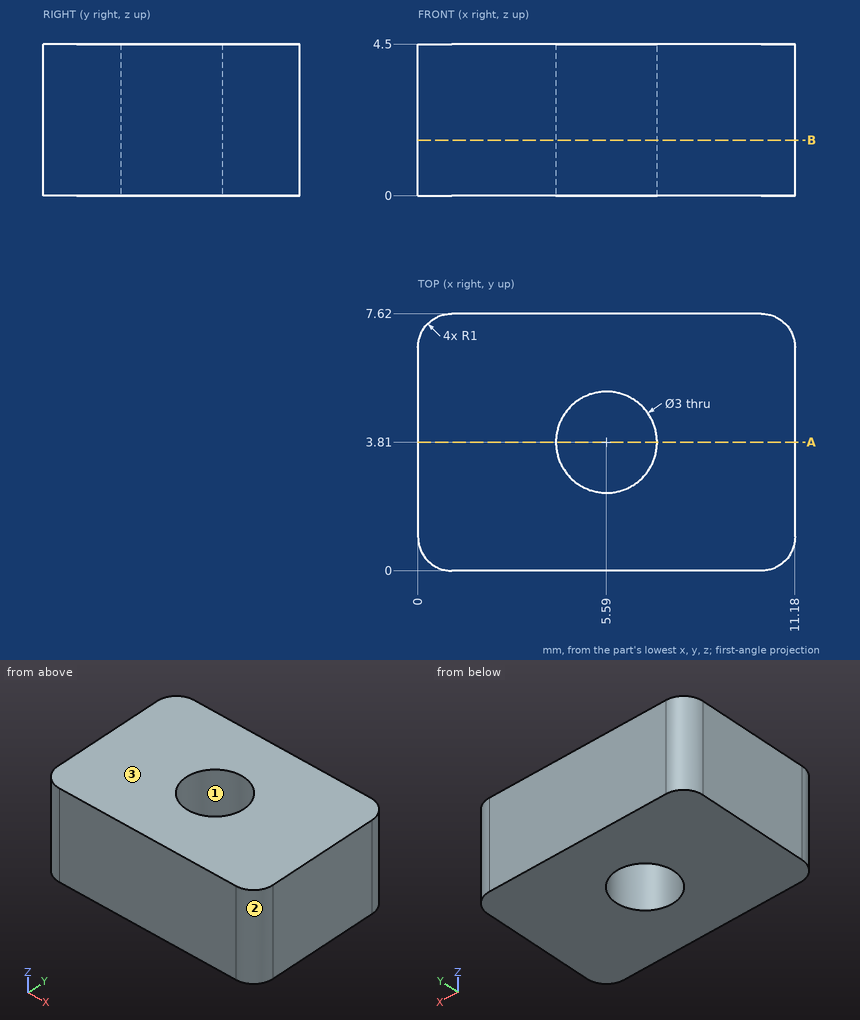
The figure shows three views and two pictorial views of one solid part (mm, origin at its lowest corner). Answer the questions. Round coordinates to 2 decimals unless told otherwise and drop trailing zeros. Loops run counter-clockwise (first coordinate to the right, second up) from the corner with the lowest first, then second, coordinate; pieces in that order, holes last. Notation, with made-up numbers: M 82.25,-30 L 122.25,-30 A23 ccw 122.25,-7 Z; hole C -36,70.25 d9. An arc over 180 degrees is marked long. Return JSON: item names as keys, results as strings.
Q1. The mould has two halves that part along Y. Classify the marked faces 1, 2 and 3: released by +Y, released by -Y, zero draft, split by the parting line, or undercut.
Results list:
{"face 1": "undercut", "face 2": "released by -Y", "face 3": "zero draft"}
Q2. Find the intervals of material crossed by line 1 along Y through (x, z) = (5.5, 4.2); line 2 along Y through (x, z) = (4.5, 1); line 3 along X through (y, z) = (5, 2.35) (1 decimal), in increasing order. Write a range as from..to.
Results list:
{"line 1": "y = 0..2.31, 5.31..7.62", "line 2": "y = 0..2.78, 4.84..7.62", "line 3": "x = 0..4.7, 6.5..11.2"}
Q3. Find section A-A, the plane y = 3.81. Determine the outline of the cut face in (x, z), plus the area to 3 significant figures.
Results list:
{"outline": "M 0,0 L 4.09,0 L 4.09,4.5 L 0,4.5 Z; M 7.09,0 L 11.18,0 L 11.18,4.5 L 7.09,4.5 Z", "area": "36.8 mm2"}
Q4. Find section B-B, the plane z = 1.65. Determine the outline of the cut face in (x, y).
Results list:
{"outline": "M 0,1 A1 ccw 1,0 L 10.18,0 A1 ccw 11.18,1 L 11.18,6.62 A1 ccw 10.18,7.62 L 1,7.62 A1 ccw 0,6.62 Z; hole C 5.59,3.81 d3"}
